Part model, mm, in its own coordinate system. A direction names the side the tool comes from. Give positions to 0.01 mm unless a question says otherwise; leave off trailing zeros. Write each loop counter-clockwise with the first axis right and the second up, starting at its lowest first coordinate (ties: lowest second). Pieces come first, ordered by that corner, then holes. Notation, with made-up numbers: M 9,43.25 L 52,43.25 A17 cw 52,72.25 Z; hole C 57,-31.5 d10. An arc over 180 degrees is marked long. Use a Markdown table: item, result. Add a question column.
from build123d import *

# Parameters (mm, degrees)
SKETCH1_R           = 46.5
SKETCH1_R_2         = 6.5
SKETCH1_R_3         = 10
SKETCH1_R_4         = 3.5
BOSS_EXTRUDE1_DEPTH = 2
SKETCH3_R           = 5
SKETCH3_R_2         = 3.5
BOSS_EXTRUDE2_DEPTH = 100
SKETCH4_R           = 30
SKETCH4_R_2         = 5
SKETCH4_R_3         = 3.5
BOSS_EXTRUDE5_DEPTH = 2
FILLET2_R           = 2
SKETCH5_R           = 1
SKETCH5_R_2         = 3.5
CUT_EXTRUDE1_DEPTH  = 1
SKETCH6_R           = 2
CUT_EXTRUDE2_DEPTH  = 2
CHAMFER2_SIZE       = 0.8
SKETCH7_R           = 61.085714235
CUT_EXTRUDE3_DEPTH  = 122.361031637


with BuildPart() as part:
    # Sketch1 → Boss-Extrude1 (new body)
    with BuildSketch(Plane(origin=(0, 0, 0), x_dir=(1, 0, 0), z_dir=(0, 1, 0))):
        with Locations(Location((0, 0, 0), (0, 0, 270))):
            Circle(SKETCH1_R)
        with Locations(Location((0, 15, 0), (0, 0, 270))):
            Circle(SKETCH1_R_2, mode=Mode.SUBTRACT)
        with Locations(Location((-12.990381057, -7.5, 0), (0, 0, 270))):
            Circle(SKETCH1_R_3, mode=Mode.SUBTRACT)
        with Locations(Location((12.990381057, -7.5, 0), (0, 0, 270))):
            Circle(SKETCH1_R_4, mode=Mode.SUBTRACT)
        with Locations(Location((0, 0, 0), (0, 0, 270))):
            Circle(SKETCH1_R_4, mode=Mode.SUBTRACT)
    extrude(amount=BOSS_EXTRUDE1_DEPTH)

    # Sketch3 → Boss-Extrude2 (add)
    with BuildSketch(Plane(origin=(0, 2, 0), x_dir=(1, 0, 0), z_dir=(0, 1, 0))):
        with Locations(Location((0, 0, 0), (0, 0, 210))):
            Circle(SKETCH3_R)
        with Locations(Location((0, 0, 0), (0, 0, 270))):
            Circle(SKETCH3_R_2, mode=Mode.SUBTRACT)
    extrude(amount=BOSS_EXTRUDE2_DEPTH)

    # Sketch6 → Cut-Extrude2 (cut)
    with BuildSketch(Plane.XZ):
        with Locations(Location((0, 35, 0), (0, 0, 270))):
            Circle(SKETCH6_R)
        with Locations(Location((27.364101886, 21.822143065, 0), (0, 0, 270))):
            Circle(SKETCH6_R)
        with Locations(Location((34.122476926, -7.788232688, 0), (0, 0, 270))):
            Circle(SKETCH6_R)
        with Locations(Location((15.185930869, -31.533910377, 0), (0, 0, 270))):
            Circle(SKETCH6_R)
        with Locations(Location((-15.185930869, -31.533910377, 0), (0, 0, 270))):
            Circle(SKETCH6_R)
        with Locations(Location((-34.122476926, -7.788232688, 0), (0, 0, 270))):
            Circle(SKETCH6_R)
        with Locations(Location((-27.364101886, 21.822143065, 0), (0, 0, 270))):
            Circle(SKETCH6_R)
    extrude(amount=-CUT_EXTRUDE2_DEPTH, mode=Mode.SUBTRACT)

    # Chamfer2
    chamfer2_edges = [part.edges().sort_by_distance(p)[0] for p in [
        (12.990381057, 0, 4),
        (34.122476926, 0, -5.788232688),
        (27.364101886, 0, 23.822143065),
        (0, 0, 37),
        (-27.364101886, 0, 23.822143065),
        (-34.122476926, 0, -5.788232688),
        (-15.185930869, 0, -29.533910377),
        (15.185930869, 0, -29.533910377),
    ]]
    chamfer(chamfer2_edges, length=CHAMFER2_SIZE)

    # Sketch7 → Cut-Extrude3 (cut, through all)
    with BuildSketch(Plane.XZ.offset(-102)):
        Circle(SKETCH7_R)
    extrude(amount=CUT_EXTRUDE3_DEPTH, mode=Mode.SUBTRACT)


with BuildPart() as body_2:
    # Sketch4 → Boss-Extrude5 (new body)
    # profile 1 of 3: a face of its own
    with BuildSketch(Plane(origin=(0, 102, 0), x_dir=(1, 0, 0), z_dir=(0, 1, 0))):
        with Locations(Location((0, 0, 0), (0, 0, 270))):
            Circle(SKETCH4_R)
        with BuildLine():
            ThreePointArc((-28.668345883, -4.373321886), (-29, 0), (-28.668345883, 4.373321886))
            ThreePointArc((-28.668345883, 4.373321886), (-14.496121896, 25.116975335), (10.555107028, 27.010918452))
            ThreePointArc((10.555107028, 27.010918452), (14.507755353, 25.110257558), (18.128572143, 22.635257278))
            ThreePointArc((18.128572143, 22.635257278), (26.141237463, 12.555305808), (29, 0))
            ThreePointArc((29, 0), (26.156181805, -12.524142821), (18.182472179, -22.591983212))
            ThreePointArc((18.182472179, -22.591983212), (14.567551204, -25.075614687), (10.619428606, -26.985695027))
            ThreePointArc((10.619428606, -26.985695027), (-14.466191914, -25.134225501), (-28.668345883, -4.373321886))
        make_face(mode=Mode.SUBTRACT)
    # profile 2 of 3: a face of its own
    with BuildSketch(Plane(origin=(0, 102, 0), x_dir=(1, 0, 0), z_dir=(0, 1, 0))):
        with BuildLine():
            ThreePointArc((0.372035902, 9.373321886), (-3.288218135, 5.713067848), (-8.288218135, 4.373321886))
            Line((-8.288218135, 4.373321886), (-28.668345883, 4.373321886))
            ThreePointArc((-28.668345883, 4.373321886), (-29, 0), (-28.668345883, -4.373321886))
            Line((-28.668345883, -4.373321886), (-8.209333805, -4.373321886))
            ThreePointArc((-8.209333805, -4.373321886), (-3.209333805, -5.713067848), (0.450920232, -9.373321886))
            Line((0.450920232, -9.373321886), (10.619428606, -26.985695027))
            ThreePointArc((10.619428606, -26.985695027), (14.567551204, -25.075614687), (18.182472179, -22.591983212))
            Line((18.182472179, -22.591983212), (7.986293771, -4.931684166))
            ThreePointArc((7.986293771, -4.931684166), (6.646547809, 0.068315834), (7.986293771, 5.068315834))
            Line((7.986293771, 5.068315834), (18.128572143, 22.635257278))
            ThreePointArc((18.128572143, 22.635257278), (14.507755353, 25.110257558), (10.555107028, 27.010918452))
            Line((10.555107028, 27.010918452), (0.372035902, 9.373321886))
        make_face()
        with Locations(Location((0, 0, 0), (0, 0, 210))):
            Circle(SKETCH4_R_2, mode=Mode.SUBTRACT)
    # profile 3 of 3: a face of its own
    with BuildSketch(Plane(origin=(0, 102, 0), x_dir=(1, 0, 0), z_dir=(0, 1, 0))):
        with Locations(Location((0, 0, 0), (0, 0, 210))):
            Circle(SKETCH4_R_2)
        with Locations(Location((0, 0, 0), (0, 0, 270))):
            Circle(SKETCH4_R_3, mode=Mode.SUBTRACT)
    extrude(amount=BOSS_EXTRUDE5_DEPTH)

    # Fillet2
    fillet2_edges = [body_2.edges().sort_by_distance(p)[0] for p in [
        (10.555107028, 103, -27.010918452),
        (-28.668345883, 103, -4.373321886),
        (18.128572143, 103, -22.635257278),
        (18.182472179, 103, 22.591983212),
        (10.619428606, 103, 26.985695027),
        (-28.668345883, 103, 4.373321886),
    ]]
    fillet(fillet2_edges, radius=FILLET2_R)

    # Sketch5 → Cut-Extrude1 (cut)
    with BuildSketch(Plane.XZ.offset(-102)):
        with Locations(Location((-15, 0, 0), (0, 0, 270))):
            Circle(SKETCH5_R)
        with Locations(Location((7.5, 12.990381057, 0), (0, 0, 270))):
            Circle(SKETCH5_R_2)
        Polygon((8.383974596, -16.52146997), (4.883974596, -10.459292144), (6.616025404, -9.459292144), (10.116025404, -15.52146997), align=None)
    extrude(amount=-CUT_EXTRUDE1_DEPTH, mode=Mode.SUBTRACT)


solid = body_2.part
1. Tool access for faces 1 (the flat face through (6.658, 102.493, -13.533)), 2 (the cylindrical face through (-14.177, 102.986, 25.298)): list every direction of +Z, -Z, +X, -X, +Y, -Y with a clear straight run to the whole face (end or side of a thin tool).
2. Drill centre lines: probe 1 along Z at (x, y) = (-16, 103.6); probe 2 along X at (y, z) = (102.1, 15.5); probe 3 along Z at (x, y) = (-13.5, 103.4). Where is each one in solid material? Low to high. Write a range as [from, to].
3. Cut at D-D (x = -5.5). Write the cut outline in (y, z).
4. Cut at C-C (x = 12.5). Write the cut outline in (y, z).
5. Cut at B-B (z = 24). Write the cut outline in (x, y), then the cut area to 3 significant figures.
6. Flat gauge pins, fed straight in: pin 1 (5 mm diameter, centred on x = -17, z = -18, fed in from -Y); pin 2 (1 mm diameter, centred on x = -15, z = 0, fed in from -Y); pin 3 (8 mm diameter, centred on x = 0, z = 0, fed in from +Y); pin 4 (0.6 mm diameter, centred on x = -13.5, y = 103, fed in from +Z). Where does each tip first touch, or does it go through?
7. Cut at A-A (x = -15). Write the cut outline in (y, z).
A:
| question | item | result |
|---|---|---|
| 1 | face 1 | -Y |
| 1 | face 2 | +Y, -Y |
| 2 | probe 1 | z = [-25.38, -24.19], [-4.37, 4.37], [24.19, 25.38] |
| 2 | probe 2 | x = [-25.69, -24.51], [3.99, 5.06], [9.94, 14.09], [24.51, 25.69] |
| 2 | probe 3 | z = [-26.79, -25.67], [-4.37, 4.37], [25.67, 26.79] |
| 3 | outline | M 102,-29.49 L 104,-29.49 L 104,-28.47 L 102,-28.47 Z; M 102,-4.77 L 104,-4.77 L 104,4.75 L 102,4.75 Z; M 102,28.47 L 104,28.47 L 104,29.49 L 102,29.49 Z |
| 4 | outline | M 102,-27.27 L 104,-27.27 L 104,-12.89 L 102,-12.89 Z; M 102,12.75 L 104,12.75 L 104,27.27 L 102,27.27 Z |
| 5 | outline | M -18,102 L -16.28,102 L -16.28,104 L -18,104 Z; M 8.9,102 L 18,102 L 18,104 L 8.9,104 Z |
| 5 | area | 21.7 mm² |
| 6 | pin 1 | passes through |
| 6 | pin 2 | stops at y = 103 |
| 6 | pin 3 | stops at y = 104 |
| 6 | pin 4 | stops at z = 26.94 |
| 7 | outline | M 102,-25.98 L 104,-25.98 L 104,-24.82 L 102,-24.82 Z; M 102,-4.37 L 104,-4.37 L 104,4.37 L 102,4.37 L 102,1 L 103,1 L 103,-1 L 102,-1 Z; M 102,24.82 L 104,24.82 L 104,25.98 L 102,25.98 Z |
